Verification items for this drawing (mm, ordinates from the low corner). A direction names the side the tool comes from. Coordinates: 2 decimals unless noted, no trailing zeros. Order: outer loops, then holes, each group sorted by start corner. A loop starts at its lowest first (then second) coordinate and runs counter-clockwise, first axis right, second up. Notation, with made-up numbers: (1, 87.25) - (38, 87.25) arc R23 ccw to (38, 125.25) - close; hole circle Ø6 at (58, 54). An arc over 180 degrees is marked (long way). Use CSV: the item, a comma, the result in double quotes. Start each with the question number.
1) Sectioned sample at D-D, the plane y = 12.5. Record the cut outline in (x, z), and give its area (3 significant figures).
2) Depth check by flat-ended pin: P1, Ø2.5, axis at x = 24.5, z = 43, coming from the -Y side; P2, Ø8, axis at x = 23, y = 7, coming from the +Z side; P3, Ø5, axis at x = 35, y = 12, coming from the +Z side; P4, Ø1, axis at x = 37, z = 39, coming from the +Y side. Enter the tip coordinate at first touch or a pass-through.
3) Draft check along Z on the marked faces 1, 2 and 3. Enter one of: released by +Z, released by -Z, zero draft, split by the parting line, or undercut.
4) Thickness scan on probe 1 along Z at (x, y) = (2, 3); probe 2 along X at (y, z) = (5, 36); probe 3 along Z at (x, y) = (27, 4.5). Record the ranges inside material, lowest first. Write a range as [from, to].
5) Sectioned sample at C-C, the plane x = 25.4. Record the cut outline in (y, z), and give its area (3 significant figures).
6) Tool access check on the marked faces 4, 5 and 6. Record the directions out of +Z, -Z, +X, -X, +Y, -Y that give a thin tool (end or side, any length) a straight path to the whole face; none if there is none.
7) Sectioned sample at A-A, the plane z = 3.81. Record the cut outline in (x, y), and give its area (3 significant figures).
8) Sectioned sample at B-B, the plane y = 6.5. Count the separate pieces of the cut face and the enclosed holes in it, and give its area (3 significant figures).
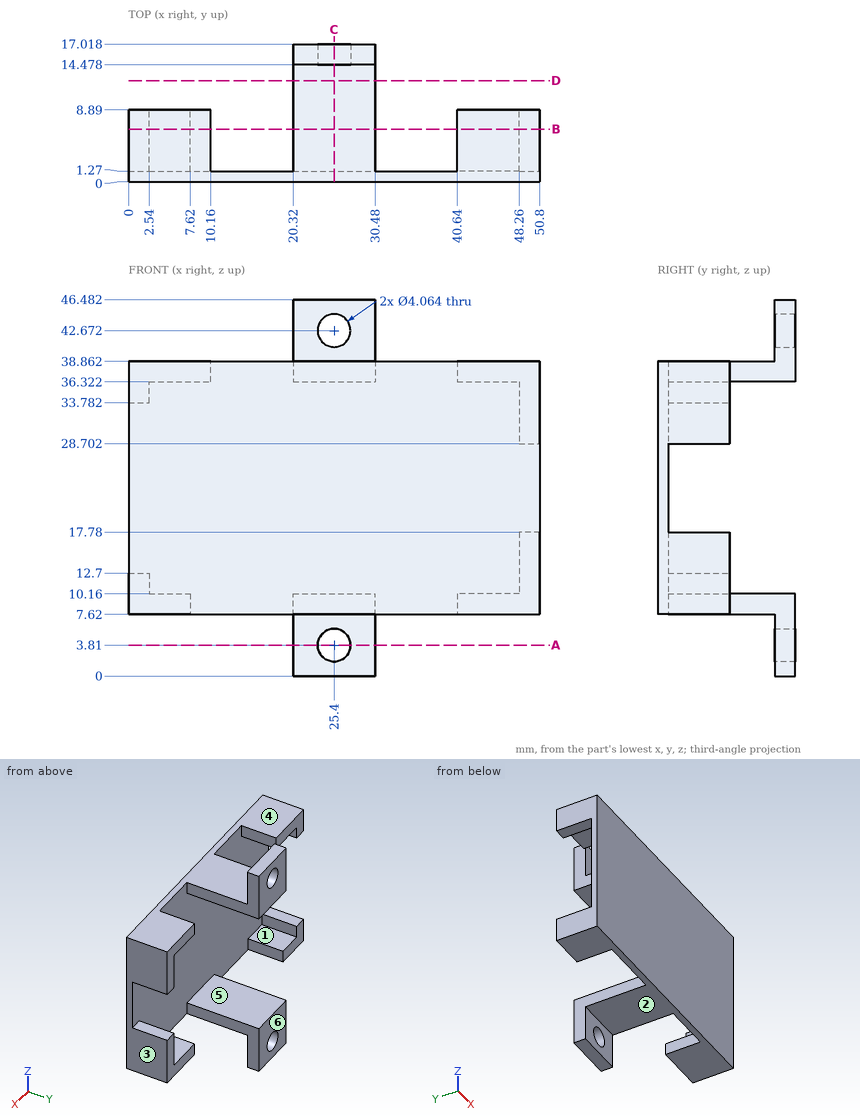
Evaluation:
1,outline,"(20.32, 7.62) - (30.48, 7.62) - (30.48, 10.16) - (20.32, 10.16) - close; (20.32, 36.32) - (30.48, 36.32) - (30.48, 38.86) - (20.32, 38.86) - close"
1,area,"51.6 mm²"
2,P1,"y = 14.48"
2,P2,"z = 38.86"
2,P3,"through"
2,P4,"y = 1.27"
3,face 1,"undercut"
3,face 2,"released by -Z"
3,face 3,"zero draft"
4,probe 1,"[7.62, 12.7], [33.78, 38.86]"
4,probe 2,"[0, 2.54], [48.26, 50.8]"
4,probe 3,"[7.62, 10.16], [36.32, 38.86]"
5,outline,"(0, 7.62) - (14.48, 7.62) - (14.48, 5.84) - (17.02, 5.84) - (17.02, 10.16) - (1.27, 10.16) - (1.27, 36.32) - (17.02, 36.32) - (17.02, 40.64) - (14.48, 40.64) - (14.48, 38.86) - (0, 38.86) - close; (14.48, 0) - (17.02, 0) - (17.02, 1.78) - (14.48, 1.78) - close; (14.48, 44.7) - (17.02, 44.7) - (17.02, 46.48) - (14.48, 46.48) - close"
5,area,"138 mm²"
6,face 4,"+Z, +X, -X, -Y"
6,face 5,"+Y"
6,face 6,"+Z, -Z, +X, -X, +Y"
7,outline,"(20.32, 14.48) - (23.37, 14.48) - (23.37, 17.02) - (20.32, 17.02) - close; (27.43, 14.48) - (30.48, 14.48) - (30.48, 17.02) - (27.43, 17.02) - close"
7,area,"15.5 mm²"
8,separate pieces,"6"
8,enclosed holes,"0"
8,area,"200 mm²"
